from build123d import *

# Parameters (mm, degrees)
ESBO_O1_W                = 31.890446896
ESBO_O1_H                = 31.890446896
ESBO_O1_W_2              = 30
ESBO_O1_H_2              = 30
RESSALTO_EXTRUS_O1_DEPTH = 149.11688245
CORTE_EXTRUS_O1_DEPTH    = 154.320238017


with BuildPart() as part:
    # Esboço1 → Ressalto-extrusão1 (new body)
    with BuildSketch(Plane.XY):
        Rectangle(ESBO_O1_W, ESBO_O1_H)
        Rectangle(ESBO_O1_W_2, ESBO_O1_H_2, mode=Mode.SUBTRACT)
    extrude(amount=RESSALTO_EXTRUS_O1_DEPTH)

    # Esboço3 → Corte-extrusão1 (cut, symmetric)
    with BuildSketch(Plane(origin=(0, 15.945223448, 0), x_dir=(1, 0, 0), z_dir=(0, 1, 0))):
        Polygon((-15.945223448, -12.692594834), (15.945223448, 0), (-15.945223448, 0), align=None)
    corte_extrus_o1 = extrude(amount=CORTE_EXTRUS_O1_DEPTH, both=True, mode=Mode.SUBTRACT)

    # Espelhar5: Corte-extrusão1 across plane
    add(corte_extrus_o1.mirror(Plane(origin=(0, 0, 74.558441225), x_dir=(1, 0, 0), z_dir=(0, 0, -1))), mode=Mode.SUBTRACT)


solid = part.part
Source: CAD feature listing. Evaluate the final solid. Frame: model axes, mm. A direction names the side the tool comes from. Coordinates: 2 decimals unless noted, no trailing zeros. Order: outer loops, then holes, each group sorted by start corner. A loop starts at its lowest first (then second) coordinate and runs counter-clockwise, first axis right, second up.
Item 1: First-contact query: P1, Ø10, axis at x = 5.5, y = -6, coming from the +Z side. Flat tip, straight axial feed; report the tip coordinate or a pass-through.
Output values:
P1: passes through
Item 2: Material intervals for line 1 (Y direction, x = 6.5, z = 100); line 2 (Z direction, x = 5, y = 15.5), sorted ascending.
Output values:
line 1: y = -15.95 to -15, 15 to 15.95
line 2: z = 4.36 to 144.76
Item 3: Cut plane C-C (z = 119). Return loops of the section in (x, y).
Output values:
outline: (-15.95, -15.95) - (15.95, -15.95) - (15.95, 15.95) - (-15.95, 15.95) - close; hole (-15, -15) - (15, -15) - (15, 15) - (-15, 15) - close
Item 4: Cut plane B-B (x = -10). Return loops of the section in (y, z).
Output values:
outline: (-15.95, 10.33) - (-15, 10.33) - (-15, 138.79) - (-15.95, 138.79) - close; (15, 10.33) - (15.95, 10.33) - (15.95, 138.79) - (15, 138.79) - close
Item 5: Set-up query: faces 4 (the face through (0, -15, 74)), 5 (the face through (-1.26, -15.28, 142.27)). Return all of +Z, -Z, +X, -X, +Y, -Y with unobstructed straight access to the full face (end or side cutting, diameter ignored); none if empty.
Output values:
face 4: +Z, -Z
face 5: +Z, -X, +Y, -Y
Item 6: Cut plane A-A (y = -5). Return loops of the section in (x, z).
Output values:
outline: (-15.95, 12.69) - (-15, 12.32) - (-15, 136.8) - (-15.95, 136.42) - close; (15, 0.38) - (15.95, 0) - (15.95, 149.12) - (15, 148.74) - close
Item 7: Pull-direction query (X, two-part tool) for faces 1 (the face through (0, 15, 74)), 2 (the face through (0, -15.945, 74)), 3 (the face through (-15.945, 0, 74)); classes: pulls with the +X half, pulls with the -X half, needs draft (parallel to the pull), parting line crosses it, or undercut.
Output values:
face 1: undercut
face 2: needs draft
face 3: pulls with the -X half
